Job drawing, mm, ordinate dimensions from the low corner. One solid piece. A direction names the side the tool comes from. Give positions to 0.01 mm unless a question says otherwise; leave off trailing zeros. Order: outer loops, then holes, each group sorted by start corner. A loop starts at its lowest first (then second) coordinate and runs counter-clockwise, first axis right, second up.
Item 1: Band-saw the part on B-B on z = 3. Give the cut face in (x, y).
Item 2: Band-saw the part on D-D on x = 7.5. Give the cut face in (y, z).
Item 3: Which spindle directions (+Z, -Z, +X, -X, +Y, -Y) get a long thin tool onto all of the face, cutting with end or side? Do the marked faces 1 and 2. Say none if no direction does.
Item 4: Wall check: L1, parallel to X at y = 16.5, z = 9.25; L2, parallel to Z at x = 2, y = 19.05; L3, parallel to Y at x = 0.75, z = 6.75. Give the ranges that are in metal, low to high.
Item 5: Band-saw the part on C-C on z = 6.35. Give the cut face in (x, y).
Item 6: Band-saw the part on A-A on y = 6.35. Give the cut face in (x, z).
Item 7: Two-plate mould, pull along Y, no slides. Class the marked faces 3, 4, 5 and 6: released by +Y, released by -Y, zero draft, split by the parting line, or undercut.
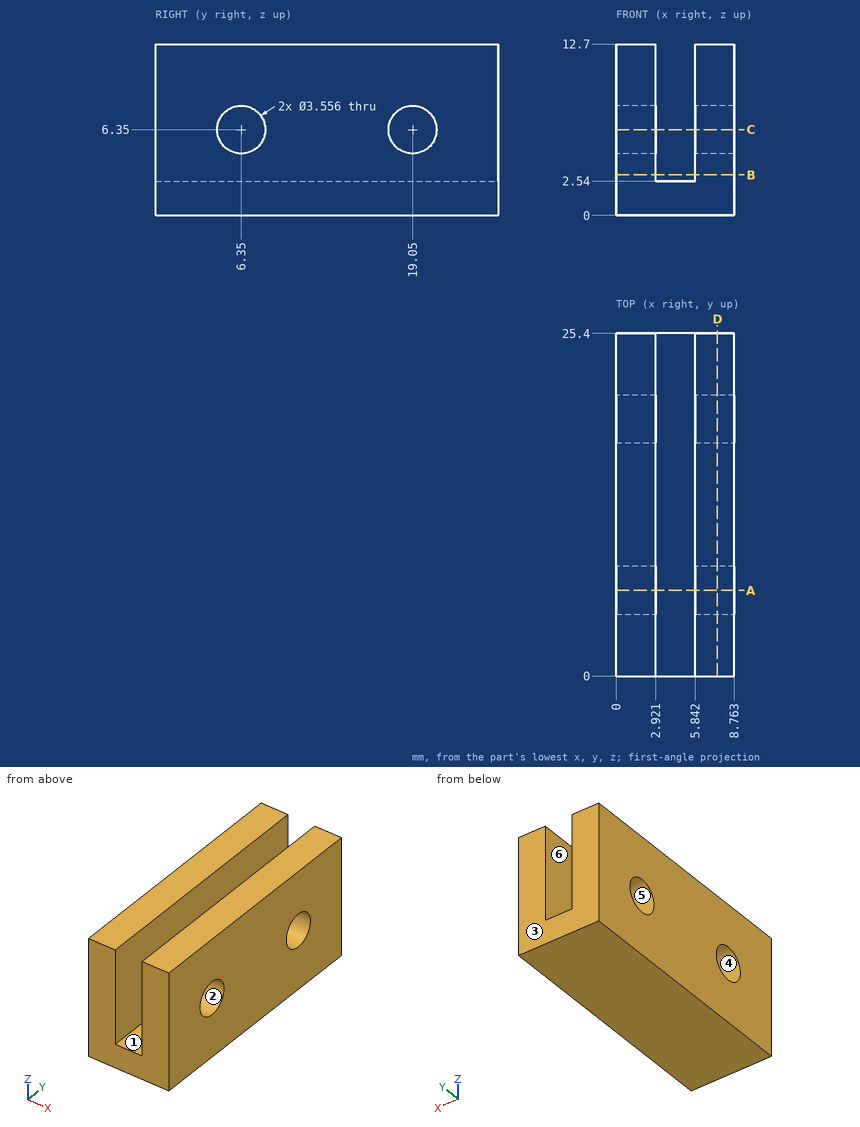
The answers:
1. outline: (0, 0) - (2.92, 0) - (2.92, 25.4) - (0, 25.4) - close; (5.84, 0) - (8.76, 0) - (8.76, 25.4) - (5.84, 25.4) - close
2. outline: (0, 0) - (25.4, 0) - (25.4, 12.7) - (0, 12.7) - close; hole circle Ø3.56 at (6.35, 6.35); hole circle Ø3.56 at (19.05, 6.35)
3. face 1: +Z, +Y, -Y
3. face 2: +X, -X
4. L1: x = 0 to 2.92, 5.84 to 8.76
4. L2: z = 0 to 4.57, 8.13 to 12.7
4. L3: y = 0 to 4.62, 8.08 to 17.32, 20.78 to 25.4
5. outline: (0, 0) - (2.92, 0) - (2.92, 4.57) - (0, 4.57) - close; (0, 8.13) - (2.92, 8.13) - (2.92, 17.27) - (0, 17.27) - close; (0, 20.83) - (2.92, 20.83) - (2.92, 25.4) - (0, 25.4) - close; (5.84, 0) - (8.76, 0) - (8.76, 4.57) - (5.84, 4.57) - close; (5.84, 8.13) - (8.76, 8.13) - (8.76, 17.27) - (5.84, 17.27) - close; (5.84, 20.83) - (8.76, 20.83) - (8.76, 25.4) - (5.84, 25.4) - close
6. outline: (0, 0) - (8.76, 0) - (8.76, 4.57) - (5.84, 4.57) - (5.84, 2.54) - (2.92, 2.54) - (2.92, 4.57) - (0, 4.57) - close; (0, 8.13) - (2.92, 8.13) - (2.92, 12.7) - (0, 12.7) - close; (5.84, 8.13) - (8.76, 8.13) - (8.76, 12.7) - (5.84, 12.7) - close
7. face 3: released by +Y
7. face 4: undercut
7. face 5: undercut
7. face 6: zero draft
